Design review of the part shown in the three views and the two pictorial views. Dimensions are in mm from the part's minimum x, y and z. Give positions to 0.01 mm unless a question says otherwise; leave off trailing zeros. Write each loop counter-clockwise with the first axis right and the second up, starting at its lowest first coordinate (ties: lowest second). Pieces come first, ordered by that corner, then holes. Notation, with made-up numbers: (-9, 41) -> (30, 41) arc R29 cw to (30, 72) -> close; hole circle Ø7 at (69, 42.25). An arc over 180 degrees is marked (long way). Return JSON: item names as keys, results as strings. Group by question number.
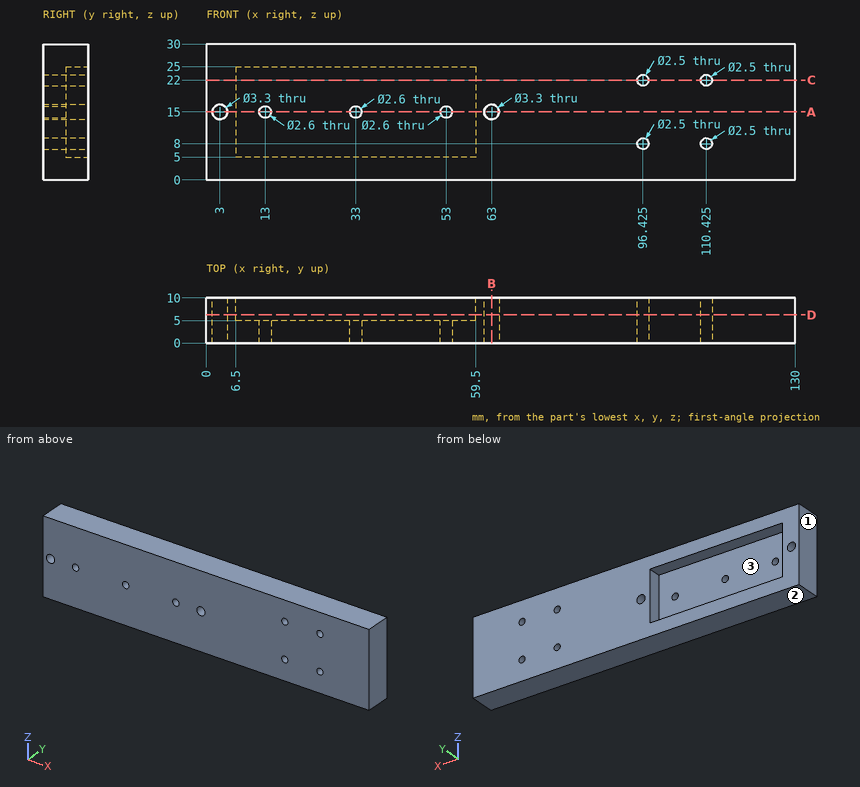
Q1. Insertion check: pin 1 (2.5 mm diameter, centred on x = 33, z = 15, fed in from -Y); pin 2 (16 mm diameter, centred on x = 34, z = 14.5, fed in from +Y). Each pin has a flat end and moves straight along its axis. Give the tip position at first contact, or say it passes through.
Q2. Take a section at D-D, the plane y = 6.25. Count the separate pieces of the cut face and the enclosed holes in it, plus the area to 3 significant figures.
Q3. For L1, parallel to X at y = 5.25, z = 22 (1 decimal); L2, parallel to X at y = 3, z = 15; L3, parallel to Z at x = 36, y = 8.25, list the stretches that pass through material, from the lowest coordinate up. Write a range as from..to.
Q4. Take a section at B-B, the plane x = 63. Give the boundary of the cut face in (y, z), plus the area to 3 significant figures.
Q5. Mouldability with a two-part tool opening along Z and no side actions: class the marked faces 1, 2 and 3 as +Z half, -Z half, draft (parallel to the pull), parting line (faces both ways), or undercut.
Q6. Take a section at A-A, the plane z = 15. Give the boundary of the cut face in (x, y), plus the area to 3 significant figures.
Q7. Take a section at C-C, the plane z = 22. Give the boundary of the cut face in (x, y) (1 decimal).
Final values:
{
 "1": {"pin 1": "passes through", "pin 2": "stops at y = 5"},
 "2": {"separate pieces": "1", "enclosed holes": "7", "area": "2,800 mm²"},
 "3": {"L1": "x = 0..6.5, 59.5..95.2, 97.7..109.2, 111.7..130", "L2": "x = 0..1.35, 4.65..11.7, 14.3..31.7, 34.3..51.7, 54.3..61.35, 64.65..130", "L3": "z = 0..5, 25..30"},
 "4": {"outline": "(0, 0) -> (10, 0) -> (10, 13.35) -> (0, 13.35) -> close; (0, 16.65) -> (10, 16.65) -> (10, 30) -> (0, 30) -> close", "area": "267 mm²"},
 "5": {"face 1": "draft", "face 2": "-Z half", "face 3": "undercut"},
 "6": {"outline": "(0, 0) -> (1.35, 0) -> (1.35, 10) -> (0, 10) -> close; (4.65, 0) -> (11.7, 0) -> (11.7, 5) -> (6.5, 5) -> (6.5, 10) -> (4.65, 10) -> close; (14.3, 0) -> (31.7, 0) -> (31.7, 5) -> (14.3, 5) -> close; (34.3, 0) -> (51.7, 0) -> (51.7, 5) -> (34.3, 5) -> close; (54.3, 0) -> (61.35, 0) -> (61.35, 10) -> (59.5, 10) -> (59.5, 5) -> (54.3, 5) -> close; (64.65, 0) -> (130, 0) -> (130, 10) -> (64.65, 10) -> close", "area": "930 mm²"},
 "7": {"outline": "(0, 0) -> (95.2, 0) -> (95.2, 10) -> (59.5, 10) -> (59.5, 5) -> (6.5, 5) -> (6.5, 10) -> (0, 10) -> close; (97.7, 0) -> (109.2, 0) -> (109.2, 10) -> (97.7, 10) -> close; (111.7, 0) -> (130, 0) -> (130, 10) -> (111.7, 10) -> close"}
}
